The listing builds one solid part. Answer for the finished solid, in the listing's coordinates (mm). A direction names the side the tool comes from. Give positions to 0.01 mm unless a question says otherwise; leave off trailing zeros. Write each loop counter-clockwise with the first axis right and the second up, starting at its lowest first coordinate (ties: lowest second). Pieces come first, ordered by that corner, then holes. Notation, with made-up numbers: (21, -38.75) -> (55, -38.75) arc R31 cw to (55, -11.75) -> close; hole circle Ø7 at (82.5, -9.75). An arc over 180 degrees is marked (long way). One line per question, with ' | ' between items.
from build123d import *

# Parameters (mm, degrees)
F0_W     = 45
F0_H     = 45
F1_DEPTH = 2
F2_W     = 40
F2_H     = 40
F2_W_2   = 35
F2_H_2   = 35
F3_DEPTH = 10
F5_START = 3
F4_W     = 41
F4_H     = 41
F4_W_2   = 35
F4_H_2   = 35
F5_DEPTH = 3
F6_R     = 5


with BuildPart() as f1:
    # F0 (on Top) → F1 (new body)
    with BuildSketch(Plane.XY):
        Rectangle(F0_W, F0_H)
    extrude(amount=F1_DEPTH)

    # F2 (on face) → F3 (join)
    with BuildSketch(Plane.XY.offset(2)):
        Rectangle(F2_W, F2_H)
        Rectangle(F2_W_2, F2_H_2, mode=Mode.SUBTRACT)
    extrude(amount=F3_DEPTH)

    # F4 (on face) → F5 (join)
    with BuildSketch(Plane.XY.offset(2).offset(F5_START)):
        Rectangle(F4_W, F4_H)
        Rectangle(F4_W_2, F4_H_2, mode=Mode.SUBTRACT)
    extrude(amount=F5_DEPTH)

    # F6
    f6_edges = [f1.edges().sort_by_distance(p)[0] for p in [
        (-22.5, 22.5, 1),
        (-20, 20, 3.5),
        (-20.5, 20.5, 6.5),
        (-20, 20, 10),
        (-22.5, -22.5, 1),
        (-20, -20, 3.5),
        (-20.5, -20.5, 6.5),
        (-20, -20, 10),
    ]]
    fillet(f6_edges, radius=F6_R)


solid = f1.part
Item 1: Find section A-A (z = 10). Write down the section's boundary in (x, y), then the cut area to 3 significant figures.
Answers below:
outline: (-20, -15) arc R5 ccw to (-15, -20) -> (20, -20) -> (20, 20) -> (-15, 20) arc R5 ccw to (-20, 15) -> close; hole (-17.5, -17.5) -> (17.5, -17.5) -> (17.5, 17.5) -> (-17.5, 17.5) -> close | area: 364 mm²
Item 2: Find section C-C (y = -13.5). Write down the section's boundary in (x, z).
Answers below:
outline: (-22.5, 0) -> (22.5, 0) -> (22.5, 2) -> (20, 2) -> (20, 5) -> (20.5, 5) -> (20.5, 8) -> (20, 8) -> (20, 12) -> (17.5, 12) -> (17.5, 2) -> (-17.5, 2) -> (-17.5, 12) -> (-20, 12) -> (-20, 8) -> (-20.5, 8) -> (-20.5, 5) -> (-20, 5) -> (-20, 2) -> (-22.5, 2) -> close
Item 3: A tool of negligible diameter and unlimited length cuts with its end or side. For faces 1 (the face through (17.5, 0, 7)), 2 (the face through (20, 0, 3)), 3 (the face through (-19.07, 19, 6.52)), 4 (the face through (2, -20, 10)), 5 (the face through (20.5, 0, 6)), from which of +Z, -Z, +X, -X, +Y, -Y can it reach the whole face along a straight path? Write none if from no direction.
Answers below:
face 1: +Z | face 2: +X, +Y, -Y | face 3: +Z, -X, +Y | face 4: +Z, +X, -X, -Y | face 5: +Z, +X, +Y, -Y
Item 4: Consider line 1 (X direction, y = 4.5, z = 5.75); line 2 (X direction, y = -15, z = 10.75). Determine where each line is inside the solid, lowest interval first. Write a range as [from, to].
Answers below:
line 1: [-20.5, -17.5], [17.5, 20.5] | line 2: [-20, -17.5], [17.5, 20]
Item 5: Determine the mould class of faces 6 (the face through (18, 0, 12)), 7 (the face through (2, 20, 10)), 8 (the face through (0, 17.5, 7)) for opening direction Y: pulls with the +Y half, pulls with the -Y half, needs draft (parallel to the pull), parting line crosses it, or undercut.
Answers below:
face 6: needs draft | face 7: pulls with the +Y half | face 8: undercut
Item 6: Flat-ended cylindrical pins translate along their axes: pin 1 (0.9 mm diameter, centred on y = 6, z = 7, fed in from -X); pin 2 (2.5 mm diameter, centred on y = 7, z = 3.5, fed in from -X); pin 3 (0.9 mm diameter, centred on x = -5, z = 4, fed in from +Y). Find the tip coordinate at first contact, or state that the pin passes through.
Answers below:
pin 1: x = -20.5 | pin 2: x = -20 | pin 3: y = 20
Item 7: Find section B-B (x = 18.5). Write down the section's boundary in (y, z).
Answers below:
outline: (-22.5, 0) -> (22.5, 0) -> (22.5, 2) -> (20, 2) -> (20, 5) -> (20.5, 5) -> (20.5, 8) -> (20, 8) -> (20, 12) -> (-20, 12) -> (-20, 8) -> (-20.5, 8) -> (-20.5, 5) -> (-20, 5) -> (-20, 2) -> (-22.5, 2) -> close
